Part print with two shaded views. Sizes in mm from the minimum x, y, z corner. Round coordinates to 2 decimals unless told otherwise and drop trailing zeros. Order: outer loops, then holes, each group sorted by start corner. A loop starts at its lowest first (then second) coordinate and runs counter-clockwise, first axis right, second up. Notation, with made-up numbers: (-3.75, -28) -> (35.25, -28) arc R35 ccw to (35.25, 5) -> close; hole circle Ø9 at (63.5, 20.25). An arc over 180 degrees is marked (long way). Answer as a JSON object with one key per item and string values.
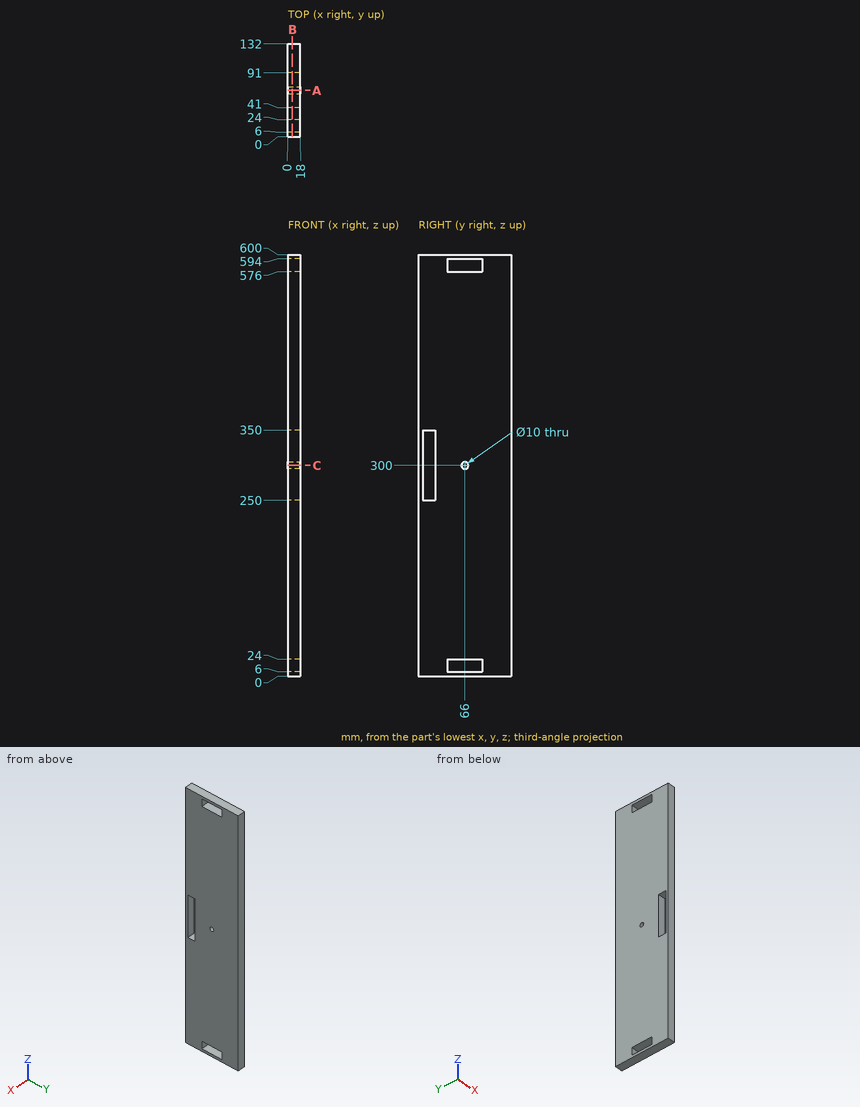
1) Cut at A-A, the plane y = 66. Give the cut face in (x, z).
Checked values:
{"outline": "(0, 0) -> (18, 0) -> (18, 6) -> (0, 6) -> close; (0, 24) -> (18, 24) -> (18, 295) -> (0, 295) -> close; (0, 305) -> (18, 305) -> (18, 576) -> (0, 576) -> close; (0, 594) -> (18, 594) -> (18, 600) -> (0, 600) -> close"}
2) Cut at C-C, the plane z = 300. Give the cut face in (x, y), plus the area to 3 significant figures.
Checked values:
{"outline": "(0, 0) -> (18, 0) -> (18, 6) -> (0, 6) -> close; (0, 24) -> (18, 24) -> (18, 61) -> (0, 61) -> close; (0, 71) -> (18, 71) -> (18, 132) -> (0, 132) -> close", "area": "1,870 mm²"}
3) Probe L1, parallel to Z at x = 1.25, y = 65; L2, parallel to Z at x = 4.5, y = 90; L3, parallel to Y at x = 13.25, z = 300. List the from-to ranges inside material, lowest first. Write a range as from..to.
Checked values:
{"L1": "z = 0..6, 24..295.1, 304.9..576, 594..600", "L2": "z = 0..6, 24..576, 594..600", "L3": "y = 0..6, 24..61, 71..132"}
4) Cut at B-B, the plane x = 6.5. Give the cut face in (y, z), plus the area to 3 significant figures.
Checked values:
{"outline": "(0, 0) -> (132, 0) -> (132, 600) -> (0, 600) -> close; hole (6, 250) -> (24, 250) -> (24, 350) -> (6, 350) -> close; hole (41, 6) -> (91, 6) -> (91, 24) -> (41, 24) -> close; hole (41, 576) -> (91, 576) -> (91, 594) -> (41, 594) -> close; hole circle Ø10 at (66, 300)", "area": "75,500 mm²"}
